Here's how the part is built. I have some questions about the finished solid (model axes, mm). Face numbers are marked on the shaded views. Round coordinates to 2 decimals unless told otherwise and drop trailing zeros. Write each loop counter-clockwise with the first axis right and the second up, starting at its lowest first coordinate (ties: lowest second). Pieces come first, ordered by that corner, then holes. Notation, with made-up numbers: (34.5, -16.5) -> (53.5, -16.5) arc R22 ccw to (53.5, 19.5) -> close; hole circle Ø7 at (37, 51). An arc over 180 degrees is marked (long way). Answer as CSV lines item,"result".
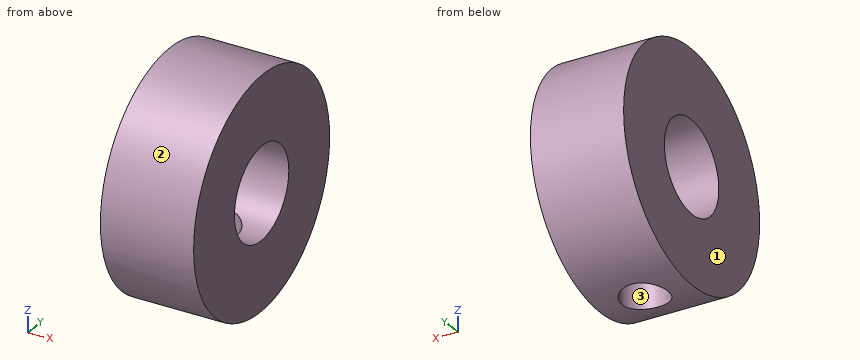
```python
from build123d import *

# Parameters (mm, degrees)
F0_R     = 63.5
F1_DEPTH = 25.4
F2_R     = 12.7
F3_DEPTH = 76.2
F4_R     = 25.4
F5_DEPTH = 31.75


with BuildPart() as f1:
    # F0 (on Right) → F1 (new body, symmetric)
    with BuildSketch(Plane.YZ):
        Circle(F0_R)
    extrude(amount=F1_DEPTH, both=True)

    # F2 (on Top) → F3 (cut)
    with BuildSketch(Plane.XY):
        Circle(F2_R)
    extrude(amount=-F3_DEPTH, mode=Mode.SUBTRACT)

    # F4 (on Right) → F5 (cut, symmetric)
    with BuildSketch(Plane.YZ):
        Circle(F4_R)
    extrude(amount=F5_DEPTH, both=True, mode=Mode.SUBTRACT)


solid = f1.part
```
1. Suppose I cut it at A-A on y = 0. Please give me the cut outline in (x, z), and give its area (3 significant figures).
Numbers:
outline,"(-25.4, -63.5) -> (-12.7, -63.5) -> (-12.7, -25.4) -> (-25.4, -25.4) -> close; (-25.4, 25.4) -> (25.4, 25.4) -> (25.4, 63.5) -> (-25.4, 63.5) -> close; (12.7, -63.5) -> (25.4, -63.5) -> (25.4, -25.4) -> (12.7, -25.4) -> close"
area,"2,900 mm^2"
2. Suppose I cut it at C-C on x = 22.5. Please give me the cut outline in (y, z).
Numbers:
outline,"circle Ø127 at (0, 0); hole circle Ø50.8 at (0, 0)"
3. Suppose I cut it at B-B on z = 0. Please give me the cut outline in (x, y).
Numbers:
outline,"(-25.4, -63.5) -> (25.4, -63.5) -> (25.4, -25.4) -> (-25.4, -25.4) -> close; (-25.4, 25.4) -> (25.4, 25.4) -> (25.4, 63.5) -> (-25.4, 63.5) -> close"
4. If I drill on line 1 (X direction, y = 0, z = -53); line 2 (Z direction, x = -14, y = 0); line 3 (Z direction, x = 17.5, y = -11.5), over which ranges is the centre line in solid material (lowest first)?
Numbers:
line 1,"x = -25.4 to -12.7, 12.7 to 25.4"
line 2,"z = -63.5 to -25.4, 25.4 to 63.5"
line 3,"z = -62.45 to -22.65, 22.65 to 62.45"
5. For pin 1 Ø8 at (x, z) = (17, -1) entering from -Y; pin 2 Ø10 at (x, y) = (9, 30) entering from +Z; pin 3 Ø12 at (x, y) = (2.5, -34.5) entering from -Z; pin 4 Ø3 at (x, y) = (-1, 0) entering from -Z, each with a flat end and sliding along its axis, tell me the tip position at first contact or that it passes through.
Numbers:
pin 1,"stops at y = -63.5"
pin 2,"stops at z = 58.37"
pin 3,"stops at z = -56.75"
pin 4,"stops at z = 25.36"
6. Suppose I cut it at D-D on z = -31.5. Please give me the cut outline in (x, y), and give its area (3 significant figures).
Numbers:
outline,"(-25.4, -55.14) -> (25.4, -55.14) -> (25.4, 55.14) -> (-25.4, 55.14) -> close; hole circle Ø25.4 at (0, 0)"
area,"5,100 mm^2"
7. If we mould it in two halves opening along Y, with no side actions, what happens to the marked faces 1, 2 and 3? For each: released by +Y, released by -Y, zero draft, split by the parting line, or undercut.
Numbers:
face 1,"zero draft"
face 2,"split by the parting line"
face 3,"undercut"
